from build123d import *

# Parameters (mm, degrees)
F0_R           = 2
F1_DEPTH       = 75
F2_W           = 3
F2_H           = 25
F3_DEPTH       = 12.5
F5_D           = 6
F5_CSINK_D     = 8
F5_CSINK_ANGLE = 90


with BuildPart() as f1:
    # F0 (on Top) → F1 (new body)
    with BuildSketch(Plane.XY):
        with BuildLine():
            Line((30, -1.5), (30, 1.5))
            Line((30, 1.5), (2.5980762114, 1.5))
            ThreePointArc((2.5980762114, 1.5), (-3, 0), (2.5980762114, -1.5))
            Line((2.5980762114, -1.5), (30, -1.5))
        make_face()
        Circle(F0_R, mode=Mode.SUBTRACT)
    extrude(amount=F1_DEPTH)

    # F2 (on Front) → F3 (cut, symmetric)
    with BuildSketch(Plane.XZ):
        with Locations((-1.5, 37.5)):
            Rectangle(F2_W, F2_H)
        with Locations((1.5, 37.5)):
            Rectangle(F2_W, F2_H)
    extrude(amount=F3_DEPTH, both=True, mode=Mode.SUBTRACT)

    # F5 (through all)
    with Locations(Plane.XZ.offset(1.5)):
        with Locations((14.9555867538, 65), (22.4555867538, 37.5), (14.9555867538, 10)):
            CounterSinkHole(F5_D / 2, F5_CSINK_D / 2, counter_sink_angle=F5_CSINK_ANGLE)


solid = f1.part
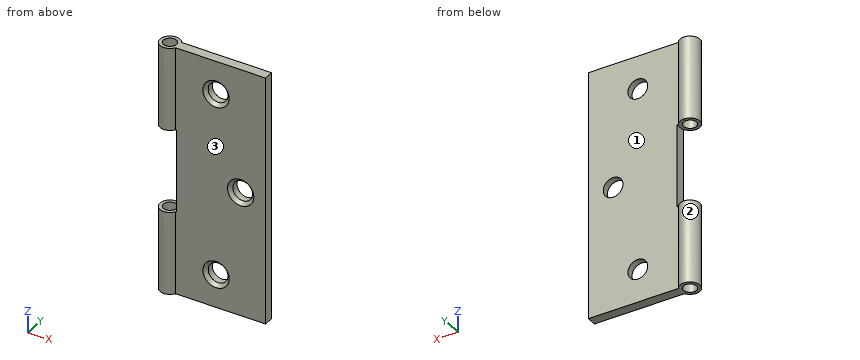
Source: CAD feature listing. Evaluate the final solid. Frame: model axes, mm. Face numbers are marked on the shaded views. A direction names the side the tool comes from. Round coordinates to 2 decimals unless told otherwise and drop trailing zeros. Loops run counter-clockwise (first coordinate to the right, second up) from the corner with the lowest first, then second, coordinate; pieces in that order, holes last.
Q1. Section D-D, the plane z = 23.5. Return loops of the section in (x, y).
Q2. First-contact query: P1, Ø1, axis at x = 15, z = 39, coming from the +Y side; P2, Ø3, axis at x = 0, y = 1, coming from the +Z side; P3, Ø12, axis at x = 15, z = 18.5, coming from the -Y side; P4, Ø1.5, axis at y = -0.5, z = 37.5, coming from the -X side. Flat tips, straight axial feed; report the tip coordinate or a pass-through.
Q3. Section C-C, the plane z = 37.5. Return loops of the section in (x, y).
Q4. Section B-B, the plane x = 0. Return loops of the section in (y, z), plus the area to 3 significant figures.
Q5. Access query for the marked faces 1, 2 and 3. Directions: +Z, -Z, +X, -X, +Y, -Y. A direction counts if a zero-diameter tool reaches every point of the face in a straight line with its end or side. Return the directions, or none.
Q6. Ray query, line 1 (X direction, y = 0.15, z = 65); line 2 (X direction, y = 0, z = 59.25); line 3 (Z direction, x = -2, y = 1.5). Return the intervals inside material, ascending.
Q7. Section A-A, the plane z = 65. Return loops of the section in (x, y).
Solutions:
1. outline: (2.6, -1.5) - (30, -1.5) - (30, 1.5) - (2.6, 1.5) arc R3 ccw (long way) to start; hole circle Ø4 at (0, 0)
2. P1: stops at y = 1.5
2. P2: stops at z = 75
2. P3: stops at y = -1.5
2. P4: stops at x = 3
3. outline: (3, -1.5) - (18.46, -1.5) - (19.46, -0.5) - (19.46, 1.5) - (3, 1.5) - close; (25.46, -0.5) - (26.46, -1.5) - (30, -1.5) - (30, 1.5) - (25.46, 1.5) - close
4. outline: (-3, 0) - (-2, 0) - (-2, 25) - (-3, 25) - close; (-3, 50) - (-2, 50) - (-2, 75) - (-3, 75) - close; (2, 0) - (3, 0) - (3, 25) - (2, 25) - close; (2, 50) - (3, 50) - (3, 75) - (2, 75) - close
4. area: 100 mm2
5. face 1: +Z, -Z, +X, +Y
5. face 2: +Z, -Z
5. face 3: +Z, -Z, +X, -Y
6. line 1: x = -3 to -1.99, 1.99 to 11.96, 17.96 to 30
6. line 2: x = -3 to -2, 2 to 30
6. line 3: z = 0 to 25, 50 to 75
7. outline: (2.6, -1.5) - (10.96, -1.5) - (11.96, -0.5) - (11.96, 1.5) - (2.6, 1.5) arc R3 ccw (long way) to start; (17.96, -0.5) - (18.96, -1.5) - (30, -1.5) - (30, 1.5) - (17.96, 1.5) - close; hole circle Ø4 at (0, 0)
